Here's how the part is built. I have some questions about the finished solid (model axes, mm). Face numbers are marked on the shaded views. A direction names the side the tool comes from. Round coordinates to 2 decimals unless told otherwise and drop trailing zeros. Order: outer loops, then holes, each group sorted by start corner. A loop starts at its lowest first (then second) coordinate and runs counter-clockwise, first axis right, second up. Notation, with made-up numbers: (-17, 83) -> (20, 83) arc R14 ccw to (20, 95) -> close; hole circle Ø1 at (49, -21.75). An arc over 180 degrees is marked (long way). Use a Markdown table: item, result. Add a question column.
from build123d import *

# Parameters (mm, degrees)
F0_W     = 107.4788756669
F0_H     = 132.3667764664
F0_W_2   = 82.2222568095
F0_H_2   = 12.9048414528
F0_H_3   = 13.0891911685
F1_DEPTH = 8.89
F2_R     = 6.5365620237
F3_DEPTH = 82.042
F4_R     = 6.3176265204
F5_DEPTH = 82.296
F6_W     = 81.5332569182
F6_H     = 22.6756446064
F6_W_2   = 82.2222568095
F6_H_2   = 20.3202562407
F7_DEPTH = 1.27
F9_D     = 11.6586
F9_DEPTH = 1.27
F9_TIP   = 3.5025968065


with BuildPart() as f1:
    # F0 (on Top) → F1 (new body)
    with BuildSketch(Plane.XY):
        with Locations((1.2904834002, -0.8295997977)):
            Rectangle(F0_W, F0_H)
        with Locations((1.7513688654, -40.0971788913)):
            Rectangle(F0_W_2, F0_H_2, mode=Mode.SUBTRACT)
        with Locations((1.7513688654, 36.1335482448)):
            Rectangle(F0_W_2, F0_H_3, mode=Mode.SUBTRACT)
    extrude(amount=F1_DEPTH)

    # F2 (on face) → F3 (join)
    with BuildSketch(Plane.YZ.offset(-39.3597595394)):
        with Locations((36.1335482448, 8.89)):
            Circle(F2_R)
    extrude(amount=F3_DEPTH)

    # F4 (on face) → F5 (join)
    with BuildSketch(Plane.YZ.offset(-39.3597595394)):
        with Locations((-40.0971788913, 8.89)):
            Circle(F4_R)
    extrude(amount=F5_DEPTH)

    # F6 (on face) → F7 (join)
    with BuildSketch(Plane.XY.offset(8.89)):
        with Locations((1.4068689197, 54.0159661323)):
            Rectangle(F6_W, F6_H)
        with Locations((1.7513688654, -23.4846300445)):
            Rectangle(F6_W_2, F6_H_2)
    extrude(amount=F7_DEPTH)

    # F9
    with Locations(Plane.XY.offset(10.16)):
        with Locations((-13.9187742025, -23.8723475486), (0, -23.5024150461), (13.735441491, -23.5012937337), (27.9312729836, -23.3157351613), (-28.114663437, -23.8734837621)):
            Hole(F9_D / 2, depth=F9_DEPTH)
            with Locations((0, 0, -(F9_DEPTH + F9_TIP / 2))):  # 118° drill point
                Cone(0, F9_D / 2, F9_TIP, mode=Mode.SUBTRACT)


solid = f1.part
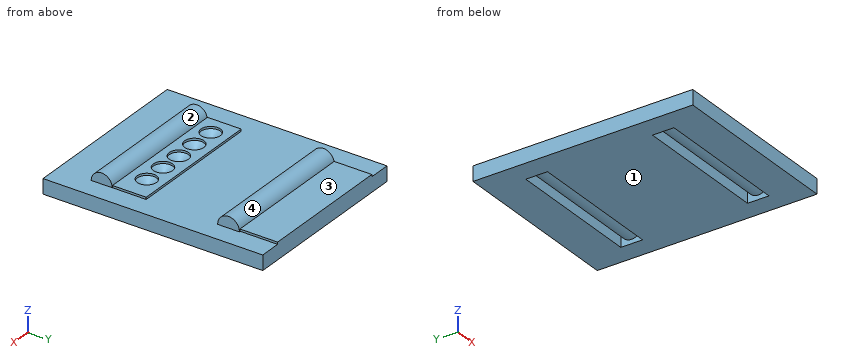
(1) On a 3-axis mill with a long thin cutter (end or side, diameter ignored), from which of +Z, -Z, +X, -X, +Y, -Y can I reach the whole of each face in a straight line? I mean the marked faces 1 and 2. Say none if no direction works.
(2) I'm going to push flat-ended pins straight in: P1, Ø1.5, axis at x = -41.5, y = -43, coming from the +Z side; P2, Ø2, axis at x = 1, y = -13.5, coming from the +Z side; P3, Ø1, axis at y = -28, z = 9.5, coming from the +X side; P4, Ø1.4, axis at y = 54.5, z = 9.5, coming from the -X side. Where does each tip first touch, or does it pass through?
(3) If we mould it in two halves opening along Y, with no side actions, what happens to the marked faces 3 and 4? For each: pulls with the +Y half, pulls with the -Y half, needs draft (parallel to the pull), parting line crosses it, or undercut.
(4) I want a section at A-A on z = 12.75. List the corners of the cut face in (x, y) for me, and give its area (3 significant figures).
(5) I want a section at B-B on x = 16. State how many separate pieces and enclosed holes the cut face has, and give its area (3 significant figures).
(6) Please list where these lines run through material, in increasing order: probe 1 along X at (y, z) = (-34.5, 0.5); probe 2 along Z at (x, y) = (40, -18.5); probe 3 along Z at (x, y) = (-42, -16.5). Write a range as from..to.
Output:
| question | item | result |
|---|---|---|
| 1 | face 1 | -Z, +X, -X, +Y, -Y |
| 1 | face 2 | none |
| 2 | P1 | z = 8.89 |
| 2 | P2 | z = 10.16 |
| 2 | P3 | x = 42.86 |
| 2 | P4 | x = -52.45 |
| 3 | face 3 | needs draft |
| 3 | face 4 | undercut |
| 4 | outline | (-39.36, -45.1) -> (42.94, -45.1) -> (42.94, -35.1) -> (-39.36, -35.1) -> close; (-39.36, 30.86) -> (42.68, 30.86) -> (42.68, 41.41) -> (-39.36, 41.41) -> close |
| 4 | area | 1,690 mm² |
| 5 | separate pieces | 5 |
| 5 | enclosed holes | 0 |
| 5 | area | 1,230 mm² |
| 6 | probe 1 | -52.45..-39.36, 42.86..55.03 |
| 6 | probe 2 | 0..10.16 |
| 6 | probe 3 | 0..8.89 |
